Geometry: final body of the model. Coordinates: model frame, mm. A direction names the side the tool comes from. Give positions to 0.01 mm unless a question says otherwise; leave off trailing zeros. Use CSV: the item, a comma, the result in double quotes. Start each with the question number.
(1) Line query: probe 1 along Z at (x, y) = (6, 4.5); probe 2 along X at (y, z) = (3.5, 14.5); probe 3 along X at (y, z) = (0, 1). Output: solid intervals per line, ascending. Write a range as [from, to].
(2) First-contact query: pin 1 Ø12 at (x, y) = (-1, 7.5) entering from -Z; pin 2 Ø1 at (y, z) = (-7, 26) entering from -X; pin 3 Ø12 at (x, z) = (-14, 24) entering from -Y; pin 4 Ø10 at (y, z) = (7, 27) entering from +X. Flat tips, straight axial feed; report the tip coordinate or a pass-through.
(3) Draft query along X for faces 1 (the flat face through (0, -5, 30)), 2 (the flat face through (1.96, 3.6, 19.35)). Return one class per face: released by +X, released by -X, zero draft, split by the parting line, or undercut.
(4) Reachability of faces 3 (the cylindrical face through (-0.338, -2.578, 5.552)), 4 (the cylindrical face through (-2.17, 9.76, 1.08)), 5 (the flat face through (2, -2, 9)) from +Z, -Z, +X, -X, +Y, -Y: full face, straight path, thin tool, end or side. Return the list, or none.
from build123d import *

# Parameters (mm, degrees)
F2_R          = 10
F3_DEPTH      = 2.2
F4_R          = 2.6
F5_DEPTH      = 27.8010001
F8_DEPTH      = 4
F8_DEPTH_BACK = 25


with BuildPart() as f1:
    # F0 (on Front) → F1 (revolve)
    with BuildSketch(Plane.XZ):
        with BuildLine():
            Line((0, 30), (0, 0))
            Line((0, 0), (18, 0))
            add(Edge.make_bspline(
                [(20, 30), (23.3665107807, 28.5300366312), (15.8290646793, 23.4868524752), (12.3142279703, 15.9642343157), (13.8468699499, 8.2686705737), (18, 0)],
                knots=[0, 0, 0, 0, 0.2654633996, 0.5684844846, 1, 1, 1, 1], degree=3))
            Line((20, 30), (0, 30))
        make_face()
    revolve(axis=Axis((0, 0, 15), (0, 0, -1)))

    # F2 (on face) → F3 (cut)
    with BuildSketch(Plane(origin=(0, 0, 0), x_dir=(1, 0, 0), z_dir=(0, 0, -1))):
        Circle(F2_R)
    extrude(amount=-F3_DEPTH, mode=Mode.SUBTRACT)

    # F4 (on face) → F5 (cut, through all)
    with BuildSketch(Plane(origin=(0, 0, 2.2), x_dir=(1, 0, 0), z_dir=(0, 0, -1))):
        Circle(F4_R)
    extrude(amount=-F5_DEPTH, mode=Mode.SUBTRACT)

    # F7 (on offset) → F8 (cut, two sides)
    with BuildSketch(Plane.XY.offset(13)) as f8_sk:
        Polygon((4.0216239956, 2.4979739332), (-0.1524968863, 4.7318155113), (-4.174120882, 2.2338415781), (-4.0216239956, -2.4979739332), (0.1524968863, -4.7318155113), (4.174120882, -2.2338415781), align=None)
    extrude(amount=-F8_DEPTH, mode=Mode.SUBTRACT)
    extrude(f8_sk.sketch, amount=F8_DEPTH_BACK, mode=Mode.SUBTRACT)


solid = f1.part
Check values:
1,probe 1,"z = [2.2, 30]"
1,probe 2,"x = [-12.87, -2.14], [2.15, 12.87]"
1,probe 3,"x = [-17.5, -10], [10, 17.5]"
2,pin 1,"stops at z = 0"
2,pin 2,"stops at x = -19.04"
2,pin 3,"stops at y = -19.05"
2,pin 4,"stops at x = 21.27"
3,face 1,"zero draft"
3,face 2,"undercut"
4,face 3,"+Z, -Z"
4,face 4,"-Z"
4,face 5,"+Z"
